from build123d import *

# Parameters (mm, degrees)
SKETCH1_W          = 42.3
SKETCH1_H          = 20
SKETCH1_W_2        = 4.6
SKETCH1_H_2        = 2.3
BASE_FLANGE1_DEPTH = 2.3
CUT_EXTRUDE1_REACH = 25.508
CUT_EXTRUDE2_REACH = 25.508
SKETCH7_W          = 0.15
SKETCH7_H          = 2.5
SKETCH8_R          = 2.5
SKETCH8_R_2        = 1
TAB1_DEPTH         = 2.3


# Sheet-metal steps are written as plain solids
with BuildPart() as part:
    # Sketch1 → Base-Flange1 (new body)
    with BuildSketch(Plane(origin=(0, 0, 0), x_dir=(1, 0, 0), z_dir=(0, 1, 0))):
        Rectangle(SKETCH1_W, SKETCH1_H)
        with Locations((-7, 0)):
            Rectangle(SKETCH1_W_2, SKETCH1_H_2, mode=Mode.SUBTRACT)
        with Locations((-2.4, -4.6)):
            Rectangle(SKETCH1_W_2, SKETCH1_H_2, mode=Mode.SUBTRACT)
        with Locations((7, 0)):
            Rectangle(SKETCH1_W_2, SKETCH1_H_2, mode=Mode.SUBTRACT)
        with Locations((-2.4, 4.6)):
            Rectangle(SKETCH1_W_2, SKETCH1_H_2, mode=Mode.SUBTRACT)
    extrude(amount=-BASE_FLANGE1_DEPTH)

    # Sketch6 → Cut-Extrude1 (cut, up to next)
    with BuildSketch(Plane(origin=(0, 0, 0), x_dir=(1, 0, 0), z_dir=(0, 1, 0)), mode=Mode.PRIVATE) as cut_extrude1_sk1:
        with BuildLine():
            Line((-18.85, 10), (-18.85, 4.45))
            Line((-18.85, 4.45), (-17.85, 4.45))
            Line((-17.85, 4.45), (-17.85, 3.45))
            Line((-17.85, 3.45), (-12.85, 3.45))
            ThreePointArc((-12.85, 3.45), (-11.435786438, 4.035786438), (-10.85, 5.45))
            Line((-10.85, 5.45), (-10.85, 6.05))
            ThreePointArc((-10.85, 6.05), (-10.264213562, 7.464213562), (-8.85, 8.05))
            Line((-8.85, 8.05), (8.85, 8.05))
            ThreePointArc((8.85, 8.05), (10.264213562, 7.464213562), (10.85, 6.05))
            Line((10.85, 6.05), (10.85, 5.45))
            ThreePointArc((10.85, 5.45), (11.435786438, 4.035786438), (12.85, 3.45))
            Line((12.85, 3.45), (17.85, 3.45))
            Line((17.85, 3.45), (17.85, 4.45))
            Line((17.85, 4.45), (18.85, 4.45))
            Line((18.85, 4.45), (18.85, 10))
            Line((18.85, 10), (-18.85, 10))
        make_face()
    cut_extrude1_tool1 = extrude(cut_extrude1_sk1.sketch, amount=-CUT_EXTRUDE1_REACH, mode=Mode.PRIVATE) & part.part
    # Sketch6 → Cut-Extrude1 (cut, up to next)
    with BuildSketch(Plane(origin=(0, 0, 0), x_dir=(1, 0, 0), z_dir=(0, 1, 0)), mode=Mode.PRIVATE) as cut_extrude1_sk2:
        with BuildLine():
            Line((18.85, -10), (-18.85, -10))
            Line((-18.85, -10), (-18.85, -4.45))
            Line((-18.85, -4.45), (-17.85, -4.45))
            Line((-17.85, -4.45), (-17.85, -3.45))
            Line((-17.85, -3.45), (-12.85, -3.45))
            ThreePointArc((-12.85, -3.45), (-11.435786438, -4.035786438), (-10.85, -5.45))
            Line((-10.85, -5.45), (-10.85, -6.05))
            ThreePointArc((-10.85, -6.05), (-10.264213562, -7.464213562), (-8.85, -8.05))
            Line((-8.85, -8.05), (8.85, -8.05))
            ThreePointArc((8.85, -8.05), (10.264213562, -7.464213562), (10.85, -6.05))
            Line((10.85, -6.05), (10.85, -5.45))
            ThreePointArc((10.85, -5.45), (11.435786438, -4.035786438), (12.85, -3.45))
            Line((12.85, -3.45), (17.85, -3.45))
            Line((17.85, -3.45), (17.85, -4.45))
            Line((17.85, -4.45), (18.85, -4.45))
            Line((18.85, -4.45), (18.85, -10))
        make_face()
    cut_extrude1_tool2 = extrude(cut_extrude1_sk2.sketch, amount=-CUT_EXTRUDE1_REACH, mode=Mode.PRIVATE) & part.part
    add(cut_extrude1_tool1.solids().sort_by_distance((15.35, 0, -3.832648))[0], mode=Mode.SUBTRACT)
    add(cut_extrude1_tool2.solids().sort_by_distance((15.35, 0, 3.832648))[0], mode=Mode.SUBTRACT)

    # Sketch7 → Cut-Extrude2 (cut, up to next)
    with BuildSketch(Plane(origin=(0, 0, 0), x_dir=(1, 0, 0), z_dir=(0, 1, 0)), mode=Mode.PRIVATE) as cut_extrude2_sk1:
        with Locations((-21.075, 7.8)):
            Rectangle(SKETCH7_W, SKETCH7_H)
    cut_extrude2_tool1 = extrude(cut_extrude2_sk1.sketch, amount=-CUT_EXTRUDE2_REACH, mode=Mode.PRIVATE) & part.part
    # Sketch7 → Cut-Extrude2 (cut, up to next)
    with BuildSketch(Plane(origin=(0, 0, 0), x_dir=(1, 0, 0), z_dir=(0, 1, 0)), mode=Mode.PRIVATE) as cut_extrude2_sk2:
        with Locations((-18.925, 7.8)):
            Rectangle(SKETCH7_W, SKETCH7_H)
    cut_extrude2_tool2 = extrude(cut_extrude2_sk2.sketch, amount=-CUT_EXTRUDE2_REACH, mode=Mode.PRIVATE) & part.part
    # Sketch7 → Cut-Extrude2 (cut, up to next)
    with BuildSketch(Plane(origin=(0, 0, 0), x_dir=(1, 0, 0), z_dir=(0, 1, 0)), mode=Mode.PRIVATE) as cut_extrude2_sk3:
        with Locations((-21.075, -7.8)):
            Rectangle(SKETCH7_W, SKETCH7_H)
    cut_extrude2_tool3 = extrude(cut_extrude2_sk3.sketch, amount=-CUT_EXTRUDE2_REACH, mode=Mode.PRIVATE) & part.part
    # Sketch7 → Cut-Extrude2 (cut, up to next)
    with BuildSketch(Plane(origin=(0, 0, 0), x_dir=(1, 0, 0), z_dir=(0, 1, 0)), mode=Mode.PRIVATE) as cut_extrude2_sk4:
        with Locations((-18.925, -7.8)):
            Rectangle(SKETCH7_W, SKETCH7_H)
    cut_extrude2_tool4 = extrude(cut_extrude2_sk4.sketch, amount=-CUT_EXTRUDE2_REACH, mode=Mode.PRIVATE) & part.part
    # Sketch7 → Cut-Extrude2 (cut, up to next)
    with BuildSketch(Plane(origin=(0, 0, 0), x_dir=(1, 0, 0), z_dir=(0, 1, 0)), mode=Mode.PRIVATE) as cut_extrude2_sk5:
        with Locations((21.075, -7.8)):
            Rectangle(SKETCH7_W, SKETCH7_H)
    cut_extrude2_tool5 = extrude(cut_extrude2_sk5.sketch, amount=-CUT_EXTRUDE2_REACH, mode=Mode.PRIVATE) & part.part
    # Sketch7 → Cut-Extrude2 (cut, up to next)
    with BuildSketch(Plane(origin=(0, 0, 0), x_dir=(1, 0, 0), z_dir=(0, 1, 0)), mode=Mode.PRIVATE) as cut_extrude2_sk6:
        with Locations((18.925, -7.8)):
            Rectangle(SKETCH7_W, SKETCH7_H)
    cut_extrude2_tool6 = extrude(cut_extrude2_sk6.sketch, amount=-CUT_EXTRUDE2_REACH, mode=Mode.PRIVATE) & part.part
    # Sketch7 → Cut-Extrude2 (cut, up to next)
    with BuildSketch(Plane(origin=(0, 0, 0), x_dir=(1, 0, 0), z_dir=(0, 1, 0)), mode=Mode.PRIVATE) as cut_extrude2_sk7:
        with Locations((21.075, 7.8)):
            Rectangle(SKETCH7_W, SKETCH7_H)
    cut_extrude2_tool7 = extrude(cut_extrude2_sk7.sketch, amount=-CUT_EXTRUDE2_REACH, mode=Mode.PRIVATE) & part.part
    # Sketch7 → Cut-Extrude2 (cut, up to next)
    with BuildSketch(Plane(origin=(0, 0, 0), x_dir=(1, 0, 0), z_dir=(0, 1, 0)), mode=Mode.PRIVATE) as cut_extrude2_sk8:
        with Locations((18.925, 7.8)):
            Rectangle(SKETCH7_W, SKETCH7_H)
    cut_extrude2_tool8 = extrude(cut_extrude2_sk8.sketch, amount=-CUT_EXTRUDE2_REACH, mode=Mode.PRIVATE) & part.part
    add(cut_extrude2_tool1.solids().sort_by_distance((-21.075, 0, -7.8))[0], mode=Mode.SUBTRACT)
    add(cut_extrude2_tool2.solids().sort_by_distance((-18.925, 0, -7.8))[0], mode=Mode.SUBTRACT)
    add(cut_extrude2_tool3.solids().sort_by_distance((-21.075, 0, 7.8))[0], mode=Mode.SUBTRACT)
    add(cut_extrude2_tool4.solids().sort_by_distance((-18.925, 0, 7.8))[0], mode=Mode.SUBTRACT)
    add(cut_extrude2_tool5.solids().sort_by_distance((21.075, 0, 7.8))[0], mode=Mode.SUBTRACT)
    add(cut_extrude2_tool6.solids().sort_by_distance((18.925, 0, 7.8))[0], mode=Mode.SUBTRACT)
    add(cut_extrude2_tool7.solids().sort_by_distance((21.075, 0, -7.8))[0], mode=Mode.SUBTRACT)
    add(cut_extrude2_tool8.solids().sort_by_distance((18.925, 0, -7.8))[0], mode=Mode.SUBTRACT)

    # Sketch8 → Tab1 (add)
    with BuildSketch(Plane(origin=(0, 0, 0), x_dir=(1, 0, 0), z_dir=(0, 1, 0))):
        with Locations((22.15, 0)):
            Circle(SKETCH8_R)
        with Locations(Location((22.15, 0, 0), (0, 0, 270))):
            Circle(SKETCH8_R_2, mode=Mode.SUBTRACT)
    extrude(amount=-TAB1_DEPTH)


solid = part.part
Geometry: final body of the model. Coordinates: model frame, mm. A direction names the side the tool comes from. Coordinates: 2 decimals unless noted, no trailing zeros. Order: outer loops, then holes, each group sorted by start corner. A loop starts at its lowest first (then second) coordinate and runs counter-clockwise, first axis right, second up.
(1) Access query for faces 1 (the face through (-17.85, -1, 4)), 2 (the face through (-21, -1, 8)), 3 (the face through (11.42, -1.13, -4.05)), 4 (the face through (-7, -1, -1.15)). Directions: +Z, -Z, +X, -X, +Y, -Y. A direction counts if a zero-diameter tool reaches every point of the face in a straight line with its end or side. Return the directions, or none.
(2) First-contact query: pin 1 (1 mm diameter, centred on y = -0.5, z = 9.5, fed in from +X); pin 2 (1 mm diameter, centred on x = 17, y = -1, fed in from -Z); pin 3 (1.2 mm diameter, centred on y = -1.5, z = 7.5, fed in from +X); pin 4 (1 mm diameter, centred on x = -15, z = 5.5, fed in from +Y). Flat tips, straight axial feed; report the tip coordinate or a pass-through.
(3) Draft query along Z for faces 5 (the face through (-10.28, -1.13, -7.45)), 6 (the face through (9.3, -1, 0)), 7 (the face through (21.15, -1, -4)). Return one class per face: pulls with the +Z half, pulls with the -Z half, needs draft (parallel to the pull), parting line crosses it, or undercut.
(4) Section query B-B (z = 0). Return the cut outline in (x, y), plus the area to 3 significant figures.
(5) Section query A-A (x = -7). Return the cut outline in (y, z), plus the area to 3 significant figures.
(6) Section query C-C (x = 22.15). Return the cut outline in (y, z).
(7) Section query D-D (y = -1.25). State how many separate pieces and enclosed holes the cut face has, plus the area to 3 significant figures.
(8) Material intervals for probe 1 along X at (y, z) = (-1.4, 0); probe 2 along Z at (x, y) = (22.15, -1.25); probe 3 along X at (y, z) = (-1.7, 6.5), sorted ascending.
Solution:
1. face 1: +Z, +Y, -Y
1. face 2: -X, +Y, -Y
1. face 3: -Z, +Y, -Y
1. face 4: +Y, -Y
2. pin 1: stops at x = 21.15
2. pin 2: stops at z = -3.45
2. pin 3: stops at x = 21
2. pin 4: passes through
3. face 5: pulls with the -Z half
3. face 6: undercut
3. face 7: needs draft
4. outline: (-21.15, -2.3) - (-9.3, -2.3) - (-9.3, 0) - (-21.15, 0) - close; (-4.7, -2.3) - (4.7, -2.3) - (4.7, 0) - (-4.7, 0) - close; (9.3, -2.3) - (21.15, -2.3) - (21.15, 0) - (9.3, 0) - close; (23.15, -2.3) - (24.65, -2.3) - (24.65, 0) - (23.15, 0) - close
4. area: 79.6 mm2
5. outline: (-2.3, -8.05) - (0, -8.05) - (0, -1.15) - (-2.3, -1.15) - close; (-2.3, 1.15) - (0, 1.15) - (0, 8.05) - (-2.3, 8.05) - close
5. area: 31.7 mm2
6. outline: (-2.3, -2.5) - (0, -2.5) - (0, -1) - (-2.3, -1) - close; (-2.3, 1) - (0, 1) - (0, 2.5) - (-2.3, 2.5) - close
7. separate pieces: 1
7. enclosed holes: 5
7. area: 522 mm2
8. probe 1: x = -21.15 to -9.3, -4.7 to 4.7, 9.3 to 21.15, 23.15 to 24.65
8. probe 2: z = -2.5 to -1, 1 to 2.5
8. probe 3: x = -21.15 to -18.85, -10.8 to 10.8, 18.85 to 21.15
